Source: CAD feature listing. Evaluate the final solid. Frame: model axes, mm. Face numbers are marked on the shaded views. Give positions to 0.01 mm unless a question says otherwise; leave off trailing zeros. Loops run counter-clockwise (first coordinate to the right, second up) from the corner with the lowest first, then second, coordinate; pieces in that order, holes last. Notation, with made-up numbers: M 75,85.5 L 134,85.5 A31 cw 134,112.5 Z; hole C -15,64 d5. An arc over 180 degrees is marked long. Answer in a Markdown table with one row per item.
```python
from build123d import *

# Parameters (mm, degrees)
SKETCH1_W           = 14
SKETCH1_H           = 14
SKETCH1_R           = 2.6
BOSS_EXTRUDE1_DEPTH = 13
CHAMFER1_SIZE       = 1


# Read off the part's stored shape, not the designer's step: M4 Tapped Hole1
with BuildPart() as part:
    # Sketch1 → Boss-Extrude1 (new body)
    with BuildSketch(Plane.XY):
        Rectangle(SKETCH1_W, SKETCH1_H)
        with Locations(Location((0, 0, 0), (0, 0, 180))):
            Circle(SKETCH1_R, mode=Mode.SUBTRACT)
    extrude(amount=BOSS_EXTRUDE1_DEPTH)

    # Chamfer1
    chamfer1_edges = [part.edges().sort_by_distance(p)[0] for p in [
        (7, 0, 13),
        (0, 7, 13),
        (-7, 0, 13),
        (0, 7, 0),
        (7, 0, 0),
        (0, -7, 0),
        (-7, 0, 0),
        (0, -7, 13),
        (-7, 7, 6.5),
        (7, 7, 6.5),
        (7, -7, 6.5),
        (-7, -7, 6.5),
    ]]
    chamfer(chamfer1_edges, length=CHAMFER1_SIZE)

    # M4 Tapped Hole1 outline → M4 Tapped Hole1 (revolve, cut)
    with BuildSketch(Plane.YX.offset(-6.5)):
        Polygon((0, 2.009055278), (1.65, 2.009055278), (1.65, 6.625), (2.025, 7), (0, 7), align=None)
    revolve(axis=Axis((0, 0, 6.5), (1, 0, 0)), mode=Mode.SUBTRACT)


solid = part.part
```
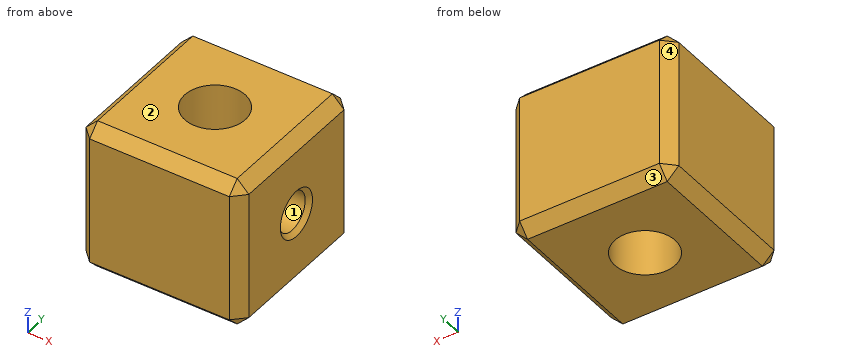
Q1. Section query D-D (x = 1.75). Output: boundary loops of the cut face in (y, z).
Values follow:
| item | result |
|---|---|
| outline | M -7,1 L -6,0 L -1.92,0 L -1.92,13 L -6,13 L -7,12 Z; M 1.92,0 L 6,0 L 7,1 L 7,12 L 6,13 L 1.92,13 Z |
Q2. Mould query, pull axis Z, two halves, no side actions, for the marked faces 1, 2, 3 and 4. Classes: +Z half, -Z half, draft (parallel to the pull), parting line (faces both ways), or undercut.
Values follow:
| item | result |
|---|---|
| face 1 | undercut |
| face 2 | +Z half |
| face 3 | -Z half |
| face 4 | draft |
Q3. Ray query, probe 1 along Z at (x, y) = (3.5, 0); probe 2 along Y at (x, z) = (0, 7.5); probe 3 along Y at (x, z) = (3, 6.5). Return the intervals inside material, ascending. Write a range as from..to.
Values follow:
| item | result |
|---|---|
| probe 1 | 0..4.85, 8.15..13 |
| probe 2 | -7..-2.6, 2.6..7 |
| probe 3 | -7..-1.65, 1.65..7 |
Q4. Section query A-A (y = 0). Output: boundary loops of the cut face in (x, z) (3 decimals), plus the area to 3 significant figures.
Values follow:
| item | result |
|---|---|
| outline | M -7,1 L -6,0 L -2.6,0 L -2.6,13 L -6,13 L -7,12 Z; M 2.6,0 L 6,0 L 7,1 L 7,4.475 L 6.625,4.85 L 2.6,4.85 Z; M 2.6,8.15 L 6.625,8.15 L 7,8.525 L 7,12 L 6,13 L 2.6,13 Z |
| area | 97.7 mm^2 |
Q5. Section query C-C (z = 6.5). Output: boundary loops of the cut face in (x, y) (3 decimals), plus the area to 3 significant figures.
Values follow:
| item | result |
|---|---|
| outline | M -7,-6 L -6,-7 L 6,-7 L 7,-6 L 7,-2.025 L 6.625,-1.65 L 2.009,-1.65 A2.6 cw long 2.009,1.65 L 6.625,1.65 L 7,2.025 L 7,6 L 6,7 L -6,7 L -7,6 Z |
| area | 157 mm^2 |
Q6. Section query B-B (x = 0). Output: boundary loops of the cut face in (y, z).
Values follow:
| item | result |
|---|---|
| outline | M -7,1 L -6,0 L -2.6,0 L -2.6,13 L -6,13 L -7,12 Z; M 2.6,0 L 6,0 L 7,1 L 7,12 L 6,13 L 2.6,13 Z |
